Autodesk Inventor part; units mm, degrees
ref_plane "YZ Plane" through (0, 0, 0) normal (1, 0, 0) x (0, 1, 0)
ref_plane "XZ Plane" through (0, 0, 0) normal (0, 1, 0) x (-1, 0, 0)
ref_plane "XY Plane" through (0, 0, 0) normal (0, 0, 1) x (1, 0, 0)
sketch "Esquisse2" plane through (0, 0, 0) normal (-1, 0, 0) x (0, 0, 1)
  circle A0 centre (0, 0) radius 8 construction
  circle A1 centre (0, 0) radius 10.5
  line L0 (0, 0) -> (5.6569, 5.6569) construction
  line L1 (0, 0) -> (8, 0) construction
  circle A2 centre (5.6569, 5.6569) radius 1.05
  circle A3 centre (-5.6569, 5.6569) radius 1.05
  circle A4 centre (-5.6569, -5.6569) radius 1.05
  circle A5 centre (5.6569, -5.6569) radius 1.05
  circle A6 centre (0, 0) radius 2
  dimension "d30" = 16
  dimension "d13" = 45
  dimension "d14" = 2.1
  dimension "d17" = 360
  dimension "d29" = 21
extrude "Extrusion5" add sketch "Esquisse2" along normal blind 5 contours A1 | A6
sketch "Esquisse6" plane through (0, 0, 0) normal (0, 1, 0) x (-1, 0, 0)
  circle A0 centre (7.5, 0) radius 3.5
  line L0 (4, 0) -> (7.5, 0)
  line L1 (10.8, 0) -> (-1.8, 0)
  line L2 (5, -10.5) -> (5, 10.5)
  point P0 (0, 0)
  point P1 (5, 0)
  point P2 (5, 2.4495)
  dimension "d46" = 7
  dimension "d48" = 1
revolve "Révolution1" cut sketch "Esquisse6" angle 360 about axis through (-4, 0, 0) along (-1, 0, 0) picked at (4.8584, 1.4572) contours L2 L0 A0
sketch "Esquisse7" plane through (0, 0, 0) normal (1, 0, 0) x (0, 0, -1)
  circle A0 centre (0, 0) radius 10.5
  circle A1 centre (-5.6569, -5.6569) radius 1.05
  circle A2 centre (5.6569, -5.6569) radius 1.05
  circle A3 centre (5.6569, 5.6569) radius 1.05
  circle A4 centre (-5.6569, 5.6569) radius 1.05
  circle A5 centre (0, 0) radius 10.5
  line L0 (0, 10.5652) -> (40, 6.1)
  line L1 (40, 6.1) -> (40, -6.1)
  line L2 (40, -6.1) -> (0, -10.5652)
  line L3 (0, -10.5652) -> (0, 10.5652)
  arc A6 (40, -6.1) -> (40, 6.1) centre (40, 0) ccw
  circle A7 centre (40, 0) radius 2.1
  line L4 (0, -14.7913) -> (0, 14.7913)
  line L5 (57.42, 0) -> (-21.82, 0)
  point P0 (1.1649, 10.4352)
  point P1 (1.1649, -10.4352)
  dimension "d49" = 40
  dimension "d53" = 4.2
  dimension "d54" = 4
extrude "Extrusion9" add sketch "Esquisse7" along normal blind 5 contours L5 L3 A0 | L5 A7 L1 L2 A0 | A0 L0 L1 A7 L5 | A0 L3 L5 | L5 A0 L3 | L3 A0 L5 | A6 L5 A7 L1 | L1 A7 L5 A6
properties part number "Biellette moteur-doigts"
CAD build for the part. Positions are in the model's coordinates, mm. A direction names the side the tool comes from. Coordinates: 2 decimals unless noted, no trailing zeros. Order: outer loops, then holes, each group sorted by start corner. A loop starts at its lowest first (then second) coordinate and runs counter-clockwise, first axis right, second up. Notation, with made-up numbers: M -36,0 L -7,0 A11 cw -7,11 Z; hole C -21,52.5 d7. An arc over 180 degrees is marked long. Write each question's results on one line, items separated by ' | '. Start each with the question number.
Q1. Cut at C-C (x = 1.25). List the corners of the cut face in (y, z).
Q2. Drill centre lines: probe 1 along Z at (x, y) = (-1.5, 4.75); probe 2 along Y at (x, z) = (1.55, -40); probe 3 along Z at (x, y) = (3.5, 0). Where is each one in solid material? Low to high. Write a range as from..to.
Q3. Pull direction Y, two halves, no side cores. Call faces 3 (the flat face through (2.465, -8.237, -20.854)), 4 (the flat face through (5, 0, -17)), 5 (the cylindrical face through (2.46, -0.09, -37.9)), 6 (the cylindrical face through (2.5, 0.1, -46.1)): +Y half, -Y half, draft (parallel to the pull), parting line (faces both ways), or undercut.
Q4. Flat gauge pins, fed straight in: P1, Ø1.3, axis at y = 5.66, z = 5.66, coming from the +X side; P2, Ø3, axis at y = -3.5, z = -14, coming from the -X side; P3, Ø1.5, axis at x = -0.5, z = -26, coming from the +Y side; P4, Ø6, axis at x = -2.5, y = -7.5, coming from the +Z side. Where does each tip first touch, or does it go through?
Q5. Which spindle directions (+Z, -Z, +X, -X, +Y, -Y) get a long thin tool onto all of the face, cutting with end or side? Do faces 1 (the cylindrical face through (0.07, 5.02, 9.22)), 2 (the flat face through (2.5, 8.3, -20.3)). Say none if no direction does.
Q6. Cut at D-D (y = -8). List the corners of the cut face in (x, z), then the cut area to 3 significant figures.
Q7. Cut at A-A (y = -1.5). List the corners of the cut face in (x, z), then the cut area to 3 significant figures.
Found:
1) outline: M -10.44,-1.16 L -6.1,-40 A6.1 ccw 6.1,-40 L 10.44,-1.16 A10.5 ccw long Z; hole C -5.66,-5.66 d2.1; hole C -5.66,5.66 d2.1; hole C 0,-40 d4.2; hole C 5.66,-5.66 d2.1; hole C 5.66,5.66 d2.1
2) probe 1: -9.36..-6.19, -5.13..5.13, 6.19..9.36 | probe 2: -6.1..-2.1, 2.1..6.1 | probe 3: -46.1..-42.1, -37.9..10.5
3) face 3: -Y half | face 4: draft | face 5: undercut | face 6: parting line
4) P1: through | P2: x = 0 | P3: y = 7.73 | P4: z = 9.49
5) face 1: -X | face 2: -Z, +X, -X, +Y
6) outline: M -5,-6.8 L 0,-6.8 L 0,-22.98 L 5,-22.98 L 5,6.8 L -5,6.8 Z | area: 217 mm²
7) outline: M -5,-10.39 L 0,-10.39 L 0,-38.53 L 5,-38.53 L 5,10.39 L -5,10.39 L -5,1.94 A3.16 cw -5,-1.94 Z; M 0,-45.91 L 5,-45.91 L 5,-41.47 L 0,-41.47 Z | area: 369 mm²
